Can you work these out from the model? Positions are in its coordinate system, mm. Face numbers are marked on the shaded views. A direction names the side the tool comes from. Round coordinates to 2 decimals unless told otherwise and drop trailing zeros. Loops run counter-clockwise (first coordinate to the right, second up) from the corner with the lowest first, then second, coordinate; pieces in that order, holes last. Notation, with made-up numbers: (50.5, -12) -> (101.5, -12) arc R23 ccw to (101.5, 22) -> close; hole circle Ø11 at (-1.5, 0.25). An arc over 180 degrees is marked (long way). Use a Markdown table: item, result.
from build123d import *

# Parameters (mm, degrees)
F0_W      = 50.8
F0_H      = 88.9
F1_DEPTH  = 63.5
F2_R      = 6.35
F3_T      = -2.54
F4_W      = 15.9004
F4_H      = 12.7
F4_R      = 3.048
F5_DEPTH  = 12.7
F6_R      = 5.08
F7_W      = 7.874
F7_H      = 4.064
F8_DEPTH  = 25.4
F9_W      = 1.27
F9_H      = 25.4
F10_DEPTH = 11.43
F11_W     = 16.129
F11_H     = 16.0528
F12_DEPTH = 13.843
F11_W_2   = 18.669
F11_H_2   = 18.5928
F13_DEPTH = 13.843
F14_W     = 3.7612880599
F14_H     = 9.271
F15_DEPTH = 13.843
F16_W     = 18.669
F16_H     = 18.5928
F17_DEPTH = 1.27
F18_W     = 7.6708
F18_H     = 15.494
F19_DEPTH = 25.4


with BuildPart() as f1:
    # F0 (on Front) → F1 (new body)
    with BuildSketch(Plane.XZ):
        Rectangle(F0_W, F0_H)
    extrude(amount=F1_DEPTH)

    # F2
    f2_edges = [f1.edges().sort_by_distance(p)[0] for p in [
        (25.4, -31.75, 44.45),
        (-25.4, -31.75, 44.45),
        (0, 0, 44.45),
        (25.4, -31.75, -44.45),
        (-25.4, -31.75, -44.45),
        (25.4, 0, 0),
        (-25.4, 0, 0),
    ]]
    fillet(f2_edges, radius=F2_R)

    # F3
    f3_openings = [f1.faces().sort_by_distance(p)[0] for p in [
        (0, -63.5, 0),
    ]]
    offset(amount=F3_T, openings=f3_openings)

    # F4 (on face) → F5 (join)
    with BuildSketch(Plane.XZ.offset(63.5)):
        with Locations((-17.4498, 21.082)):
            Rectangle(F4_W, F4_H)
        with Locations((-17.4498, 21.082)):
            Circle(F4_R, mode=Mode.SUBTRACT)
        with Locations((17.4498, 21.082)):
            Rectangle(F4_W, F4_H)
        with Locations((17.4498, 21.082)):
            Circle(F4_R, mode=Mode.SUBTRACT)
    extrude(amount=-F5_DEPTH)

    # F6
    f6_edges = [f1.edges().sort_by_distance(p)[0] for p in [
        (-9.4996, -57.15, 27.432),
        (-9.4996, -57.15, 14.732),
        (9.4996, -57.15, 14.732),
        (9.4996, -57.15, 27.432),
        (-22.86, -57.15, 27.432),
        (22.86, -57.15, 27.432),
        (-22.86, -57.15, 14.732),
        (22.86, -57.15, 14.732),
    ]]
    fillet(f6_edges, radius=F6_R)

    # F7 (on face) → F8 (cut)
    with BuildSketch(Plane.XY.offset(44.45)):
        with Locations((0, -10.16)):
            Rectangle(F7_W, F7_H)
    extrude(amount=-F8_DEPTH, mode=Mode.SUBTRACT)

    # F9 (on face) → F10 (join)
    with BuildSketch(Plane.XZ.offset(2.54)):
        with Locations((-9.525, 25.4)):
            Rectangle(F9_W, F9_H)
        with Locations((9.525, 25.4)):
            Rectangle(F9_W, F9_H)
    extrude(amount=F10_DEPTH)

    # F11 (on face) → F12 (cut)
    with BuildSketch(Plane(origin=(0, 0, 0), x_dir=(-1, 0, 0), z_dir=(0, 1, 0))):
        with Locations((0, -35.1536)):
            Rectangle(F11_W, F11_H)
    extrude(amount=-F12_DEPTH, mode=Mode.SUBTRACT)

    # F11 (on face) → F13 (join)
    with BuildSketch(Plane(origin=(0, 0, 0), x_dir=(-1, 0, 0), z_dir=(0, 1, 0))):
        with Locations((0, -35.1536)):
            Rectangle(F11_W_2, F11_H_2)
        with Locations((0, -35.1536)):
            Rectangle(F11_W, F11_H, mode=Mode.SUBTRACT)
    extrude(amount=-F13_DEPTH)

    # F14 (on face) → F15 (cut)
    with BuildSketch(Plane(origin=(0, 0, 0), x_dir=(-1, 0, 0), z_dir=(0, 1, 0))):
        with Locations((-7.45385597, -35.1536)):
            Rectangle(F14_W, F14_H)
    extrude(amount=-F15_DEPTH, mode=Mode.SUBTRACT)

    # F16 (on face) → F17 (join)
    with BuildSketch(Plane.XZ.offset(13.843)):
        with Locations((0, -35.1536)):
            Rectangle(F16_W, F16_H)
    extrude(amount=F17_DEPTH)

    # F18 (on face) → F19 (cut)
    with BuildSketch(Plane(origin=(-25.4, 0, 0), x_dir=(0, -1, 0), z_dir=(-1, 0, 0))):
        with Locations((51.2709531141, -24.9448278919)):
            Rectangle(F18_W, F18_H)
    extrude(amount=-F19_DEPTH, mode=Mode.SUBTRACT)


solid = f1.part
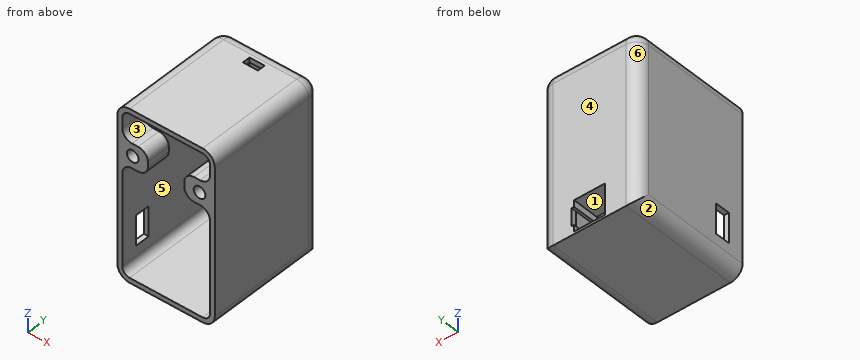
1. Which directions (+Z, -Z, +X, -X, +Y, -Y) give clear straight access to the entire face, cutting with the end or side of a thin tool? Please do the marked faces 1, 2 and 3.
Answer sheet:
| item | result |
|---|---|
| face 1 | +Y |
| face 2 | -Z, -X, +Y, -Y |
| face 3 | -Y |
2. I want a section at D-D (y = -59). State how many separate pieces and enclosed holes the cut face has, plus the area to 3 significant figures.
Answer sheet:
| item | result |
|---|---|
| separate pieces | 1 |
| enclosed holes | 3 |
| area | 943 mm² |
3. Will these pins go through, and if not, where does the flat tip stop? pin 1 Ø17.5 at (x, z) = (0, -31) entering from -Y; pin 2 Ø3.5 at (y, z) = (-7, -42.5) entering from -X; pin 3 Ø0.6 at (x, z) = (-9.5, 27) entering from -Y.
Answer sheet:
| item | result |
|---|---|
| pin 1 | stops at y = -15.11 |
| pin 2 | stops at x = -24.82 |
| pin 3 | stops at y = -13.97 |
4. I want a section at A-A (x = -1). Please give me the cut outline in (y, z).
Answer sheet:
| item | result |
|---|---|
| outline | (-63.5, -44.45) -> (0, -44.45) -> (0, -43.18) -> (-13.84, -43.18) -> (-13.84, -27.13) -> (0, -27.13) -> (0, 38.1) arc R6.35 ccw to (-6.35, 44.45) -> (-8.13, 44.45) -> (-8.13, 41.91) -> (-6.35, 41.91) arc R3.81 cw to (-2.54, 38.1) -> (-2.54, -25.86) -> (-15.11, -25.86) -> (-15.11, -41.91) -> (-63.5, -41.91) -> close; (-63.5, 41.91) -> (-12.19, 41.91) -> (-12.19, 44.45) -> (-63.5, 44.45) -> close |
5. I need wall thicknesses on line 1 (Z direction, x = -8, y = -11); line 2 (X direction, y = -10, z = 33.5); line 3 (X direction, y = -32.5, z = 11.5). Which ranges of each line are inside material? Lowest first, please.
Answer sheet:
| item | result |
|---|---|
| line 1 | z = -44.45 to -43.18, -27.13 to -25.86, 41.91 to 44.45 |
| line 2 | x = -25.4 to -22.86, -10.16 to -8.89, 8.89 to 10.16, 22.86 to 25.4 |
| line 3 | x = -25.4 to -22.86, 22.86 to 25.4 |
6. I want a section at C-C (z = -11). Please give me the cut outline in (x, y).
Answer sheet:
| item | result |
|---|---|
| outline | (-25.4, -63.5) -> (-22.86, -63.5) -> (-22.86, -6.35) arc R3.81 cw to (-19.05, -2.54) -> (19.05, -2.54) arc R3.81 cw to (22.86, -6.35) -> (22.86, -63.5) -> (25.4, -63.5) -> (25.4, -6.35) arc R6.35 ccw to (19.05, 0) -> (-19.05, 0) arc R6.35 ccw to (-25.4, -6.35) -> close |
7. If we mould it in two halves opening along X, with no side actions, what happens to the marked faces 4, 5 and 6? For each: +X half, -X half, draft (parallel to the pull), parting line (faces both ways), or undercut.
Answer sheet:
| item | result |
|---|---|
| face 4 | draft |
| face 5 | undercut |
| face 6 | -X half |
8. I want a section at B-B (y = -24). Please give me the cut outline in (x, z), plus the area to 3 significant figures.
Answer sheet:
| item | result |
|---|---|
| outline | (-25.4, -38.1) arc R6.35 ccw to (-19.05, -44.45) -> (19.05, -44.45) arc R6.35 ccw to (25.4, -38.1) -> (25.4, 38.1) arc R6.35 ccw to (19.05, 44.45) -> (-19.05, 44.45) arc R6.35 ccw to (-25.4, 38.1) -> close; hole (-22.86, -38.1) arc R3.81 ccw to (-19.05, -41.91) -> (19.05, -41.91) arc R3.81 ccw to (22.86, -38.1) -> (22.86, 38.1) arc R3.81 ccw to (19.05, 41.91) -> (-19.05, 41.91) arc R3.81 ccw to (-22.86, 38.1) -> close |
| area | 662 mm² |
